Check sheet for the modelled part. Datum: model origin and axes. Units: mm. A direction names the side the tool comes from. Round coordinates to 2 decimals unless told otherwise and drop trailing zeros. Loops run counter-clockwise (first coordinate to the right, second up) from the corner with the lowest first, then second, coordinate; pieces in that order, holes last. Notation, with made-up numbers: (59, 39) - (114, 39) arc R18 ccw to (114, 59) - close; hole circle Ø1 at (-1.5, -10). An arc over 180 degrees is marked (long way). Answer in a Markdown table with one row per item. Add a question column.
(1) Cross-section at A-A on z = 7.75. Enter the section's corners in (x, y).
(2) Gauge pin test, flat ends, axial feed: pin 1 (10 mm diameter, centred on x = 10.5, z = 9, fed in from +Y); pin 2 (10.5 mm diameter, centred on y = 11.5, z = 15, fed in from -X); pin 3 (5 mm diameter, centred on y = -12, z = 14.5, fed in from +X); pin 4 (2.5 mm diameter, centred on x = 18.51, y = 8.23, fed in from -Z). Record the tip position at first contact, or that the pin passes through.
(3) Thickness scan on line 1 along Y through (x, z) = (0, 13.5); line 2 along Z through (x, y) = (9, 10); line 3 along X through (y, z) = (12, 18.5) (3 decimals). Record the ranges inside material, lowest first.
(4) Access from +Z, -Z, +X, -X, +Y, -Y to the whole of each face (thin tool, end or side, straight path). Record for faces 4 (the flat face through (-13.94, -3.2, 13.69)), 5 (the cylindrical face through (-17.86, 11.98, 2.54)), 6 (the flat face through (-8.899, -11.385, 13.688)), 7 (the flat face through (22.21, 5.73, 7.54)), 8 (the cylindrical face through (15.132, 6.371, 7.535)).
(5) Cross-section at B-B on z = 12. Enter the section's corners in (x, y) (3 decimals).
(6) Cross-section at C-C on z = 2.5. Enter the section's corners in (x, y), then the cut area to 3 significant figures.
(7) Mould release check, pull along Y, two halves, no side actions. Record for faces 1 (the flat face through (4.805, 13, 14)), 2 (the cylindrical face through (0.106, 24.022, 13.521)), 3 (the cylindrical face through (-0.506, 16.941, 13.863)): +Y half, -Y half, draft (parallel to the pull), parting line (faces both ways), or undercut.
from build123d import *

# Parameters (mm, degrees)
PAD_DEPTH          = 10
POCKET_DEPTH       = 5
SKETCH002_R        = 1.481767
POCKET001_DEPTH    = 5
POLARPATTERN_COUNT = 3
SKETCH003_R        = 2.332395
PAD001_DEPTH       = 10


with BuildPart() as part:
    # Sketch → Pad (new body)
    with BuildSketch(Plane.XY):
        Polygon((13.856406, -24), (27.712813, 0), (13.856406, 24), (-13.856406, 24), (-27.712813, 0), (-13.856406, -24), align=None)
    extrude(amount=PAD_DEPTH)

    # Sketch001 (on Face8 of Pad) → Pocket (cut)
    with BuildSketch(Plane.XY.offset(10)):
        with BuildLine():
            ThreePointArc((-18.488317, 8.556219), (-13.038939, 9.994402), (-14.477122, 15.443781))
            Line((-14.477122, 15.443781), (-28.403704, 23.554379))
            ThreePointArc((-28.403704, 23.554379), (-33.853083, 22.116196), (-32.4149, 16.666817))
            Line((-32.4149, 16.666817), (-18.488317, 8.556219))
        make_face()
    pocket = extrude(amount=-POCKET_DEPTH, mode=Mode.SUBTRACT)

    # Sketch002 (on Face12 of Pocket) → Pocket001 (cut)
    with BuildSketch(Plane.XY.offset(5)):
        with Locations((-16.379377, 11.911345)):
            Circle(SKETCH002_R)
    pocket001 = extrude(amount=-POCKET001_DEPTH, mode=Mode.SUBTRACT)

    # PolarPattern: Pocket001, Pocket ×3 about axis
    polarpattern_axis = Axis((0, 0, 5), (0, 0, 1))
    for i in range(1, POLARPATTERN_COUNT):
        add(pocket001.rotate(polarpattern_axis, i * 360 / POLARPATTERN_COUNT), mode=Mode.SUBTRACT)
        add(pocket.rotate(polarpattern_axis, i * 360 / POLARPATTERN_COUNT), mode=Mode.SUBTRACT)

    # Sketch003 (on Face5 of PolarPattern) → Pad001 (join)
    with BuildSketch(Plane.XY.offset(10)):
        with BuildLine():
            ThreePointArc((-4.035282, -8.27825), (0.242823, -9.206191), (4.466063, -8.054017))
            Line((4.466063, -8.054017), (14.220197, -13.581932))
            ThreePointArc((14.220197, -13.581932), (20.76966, -11.770691), (18.958419, -5.221228))
            Line((18.958419, -5.221228), (9.204285, 0.306686))
            ThreePointArc((9.204285, 0.306686), (7.957073, 4.636583), (4.805, 7.856519))
            Line((4.805, 7.856519), (4.805, 19.21837))
            ThreePointArc((4.805, 19.21837), (0, 24.02337), (-4.805, 19.21837))
            Line((-4.805, 19.21837), (-4.805, 7.856519))
            ThreePointArc((-4.805, 7.856519), (-8.076559, 4.425168), (-9.207654, -0.178949))
            Line((-9.207654, -0.178949), (-18.801422, -6.305717))
            ThreePointArc((-18.801422, -6.305717), (-20.264886, -12.941553), (-13.62905, -14.405017))
            Line((-13.62905, -14.405017), (-4.035282, -8.27825))
        make_face()
        with Locations((0, 19.21837)):
            Circle(SKETCH003_R, mode=Mode.SUBTRACT)
        with Locations((-16.215236, -10.355367)):
            Circle(SKETCH003_R, mode=Mode.SUBTRACT)
        with Locations((16.589308, -9.40158)):
            Circle(SKETCH003_R, mode=Mode.SUBTRACT)
    extrude(amount=PAD001_DEPTH)

    # Sketch005 → Groove (revolve, cut)
    with BuildSketch(Plane.YZ):
        Polygon((0, 21.841362), (31.185255, 14.444732), (30.454723, 21.841362), align=None)
    revolve(axis=Axis((0, 0, 0), (0, 0, 1)), mode=Mode.SUBTRACT)


solid = part.part
Answers:
| question | item | result |
|---|---|---|
| 1 | outline | (-27.71, 0) - (-13.86, -24) - (-6.15, -24) - (-6.14, -20.26) arc R3.99 cw to (1.83, -20.29) - (1.82, -24) - (13.86, -24) - (27.71, 0) - (23.86, 6.67) - (20.61, 4.82) arc R3.99 cw to (16.65, 11.73) - (19.87, 13.58) - (13.86, 24) - (-13.86, 24) - (-17.71, 17.33) - (-14.48, 15.44) arc R3.99 cw to (-18.49, 8.56) - (-21.69, 10.42) - close |
| 2 | pin 1 | stops at y = 24 |
| 2 | pin 2 | stops at x = -22 |
| 2 | pin 3 | stops at x = 21.39 |
| 2 | pin 4 | passes through |
| 3 | line 1 | y = -9.21 to 16.89, 21.55 to 24.02 |
| 3 | line 2 | z = 0 to 10 |
| 3 | line 3 | x = -4.805 to 4.805 |
| 4 | face 4 | +Z, -X, +Y |
| 4 | face 5 | +Z, -Z |
| 4 | face 6 | +Z, -Y |
| 4 | face 7 | +Z, +Y |
| 4 | face 8 | +Z |
| 5 | outline | (-18.801, -6.306) arc R4.805 ccw to (-13.629, -14.405) - (-4.035, -8.278) arc R9.209 ccw to (4.466, -8.054) - (14.22, -13.582) arc R4.805 ccw to (18.958, -5.221) - (9.204, 0.307) arc R9.209 ccw to (4.805, 7.857) - (4.805, 19.218) arc R4.805 ccw to (-4.805, 19.218) - (-4.805, 7.857) arc R9.209 ccw to (-9.208, -0.179) - close; hole circle Ø4.665 at (-16.215, -10.355); hole circle Ø4.665 at (0, 19.218); hole circle Ø4.665 at (16.589, -9.402) |
| 6 | outline | (-27.71, 0) - (-13.86, -24) - (13.86, -24) - (27.71, 0) - (13.86, 24) - (-13.86, 24) - close; hole circle Ø2.96 at (-16.38, 11.91); hole circle Ø2.96 at (-2.13, -20.14); hole circle Ø2.96 at (18.51, 8.23) |
| 6 | area | 1,970 mm^2 |
| 7 | face 1 | draft |
| 7 | face 2 | +Y half |
| 7 | face 3 | undercut |
